Verification items for the finished model (mm, model axes). Coordinates: 2 decimals unless noted, no trailing zeros. Order: outer loops, then holes, each group sorted by start corner. A loop starts at its lowest first (then second) coordinate and runs counter-clockwise, first axis right, second up. Notation, with made-up numbers: M 7,62.5 L 66,62.5 A28 ccw 66,96.5 Z; hole C -20,-8 d2. An arc over 180 degrees is marked long. Return JSON: item names as keys, results as strings. Group by question number.
Q1. Section check B-B, the plane x = 27. Enter the section's corners in (y, z), then the cut area to 3 significant figures.
Q2. Go/stop test with a flat-tipped pin: pin 1 Ø5 at (x, z) = (23.5, -13.5) entering from +Y. Record where the tip stops, or that it passes through.
Q3. Section check C-C, the plane y = -12.7. Enter the section's corners in (x, z), then the cut area to 3 significant figures.
Q4. Thickness scan on probe 1 along Z at (x, y) = (0, -8); probe 2 along Z at (x, y) = (-13.5, -1.5); probe 3 along X at (y, z) = (-18.5, 3). Record the ranges inside material, lowest first.
Q5. Section check A-A, the plane z = 0. Enter the section's corners in (x, y).
Q6. Mould release check, pull along Z, two halves, no side actions. Record for faces 1 (the face through (-2, -13, -41.757)), 2 (the face through (21.938, -12.522, -9.096)), 3 (the face through (-26.047, -12.543, -4.191)): pulls with the +Z half, pulls with the -Z half, needs draft (parallel to the pull), parting line crosses it, or undercut.
Q7. Section check D-D, the plane z = -26.5. Enter the section's corners in (x, y).
from build123d import *

# Parameters (mm, degrees)
F0_W     = 95.25
F0_H     = 76.2
F0_R     = 23.749
F1_DEPTH = 25.4
F3_D     = 7.1374


with BuildPart() as f1:
    # F0 (on Front) → F1 (new body)
    with BuildSketch(Plane.XZ):
        with Locations((-0.95523, -3.657167)):
            Rectangle(F0_W, F0_H)
        Circle(F0_R, mode=Mode.SUBTRACT)
    extrude(amount=F1_DEPTH)

    # F3 (through all)
    with Locations(Plane.XY.offset(34.442833)):
        with Locations((-29.612565, -12.7), (26.31861, -12.7)):
            Hole(F3_D / 2)


solid = f1.part
Numbers:
{
 "1": {"outline": "M -25.4,-41.76 L -16.2,-41.76 L -16.2,34.44 L -25.4,34.44 Z; M -9.2,-41.76 L 0,-41.76 L 0,34.44 L -9.2,34.44 Z", "area": "1,400 mm2"},
 "2": {"pin 1": "stops at y = 0"},
 "3": {"outline": "M -48.58,-41.76 L -33.18,-41.76 L -33.18,34.44 L -48.58,34.44 Z; M -26.04,-41.76 L 22.75,-41.76 L 22.75,-6.82 A23.75 cw long 22.75,6.82 L 22.75,34.44 L -26.04,34.44 Z; M 29.89,-41.76 L 46.67,-41.76 L 46.67,34.44 L 29.89,34.44 Z", "area": "4,410 mm2"},
 "4": {"probe 1": "z = -41.76 to -23.75, 23.75 to 34.44", "probe 2": "z = -41.76 to -19.54, 19.54 to 34.44", "probe 3": "x = -48.58 to -23.56, 23.56 to 46.67"},
 "5": {"outline": "M -48.58,-25.4 L -23.75,-25.4 L -23.75,0 L -48.58,0 Z; M 23.75,-25.4 L 46.67,-25.4 L 46.67,0 L 23.75,0 L 23.75,-10.22 A3.57 cw long 23.75,-15.18 Z; hole C -29.61,-12.7 d7.14"},
 "6": {"face 1": "pulls with the -Z half", "face 2": "undercut", "face 3": "needs draft"},
 "7": {"outline": "M -48.58,-25.4 L 46.67,-25.4 L 46.67,0 L -48.58,0 Z; hole C -29.61,-12.7 d7.14; hole C 26.32,-12.7 d7.14"}
}
